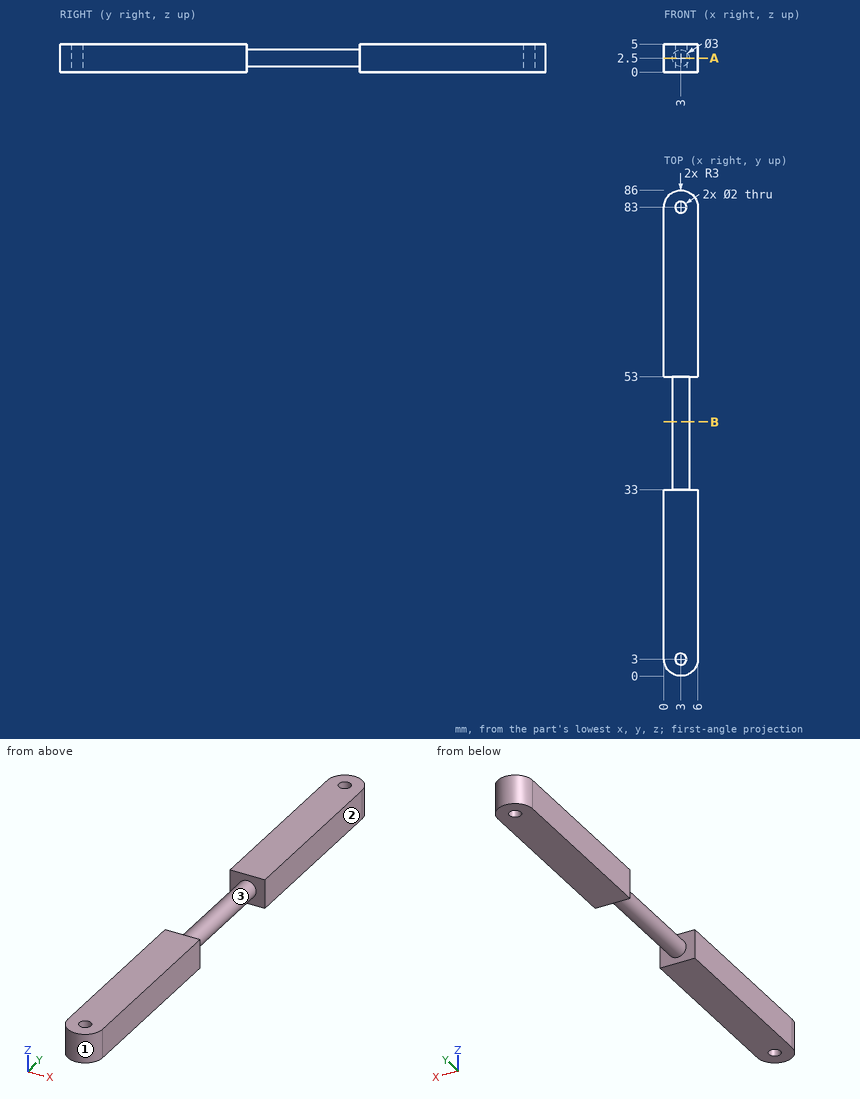
Print and shaded views of the part. All mm, measured from the part's lowest x, y and z. Coordinates: 2 decimals unless noted, no trailing zeros. Loops run counter-clockwise (first coordinate to the right, second up) from the corner with the lowest first, then second, coordinate; pieces in that order, holes last. Notation, with made-up numbers: (46, 62.25) -> (54, 62.25) arc R20 ccw to (54, 72.25) -> close; hole circle Ø9 at (56.25, 14.5). An arc over 180 degrees is marked (long way). Use a Markdown table: item, result. Add a question column.
Item 1: Probe probe 1 along Y at (x, z) = (3, 2.85); probe 2 along Y at (x, z) = (2.9, 4.5); probe 3 along X at (y, z) = (83, 2.15). List the from-to ranges inside material, lowest first.
Item 2: Band-saw the part on B-B on y = 45. Write the cut outline in (x, z), plus the area to 3 significant figures.
Item 3: Flat gauge pins, fed straight in: P1, Ø2, axis at x = 5, z = 2.5, coming from the +Y side; P2, Ø1.5, axis at x = 4, z = 1.5, coming from the -Y side. Where does each tip first touch, or does it go through?
Item 4: Band-saw the part on A-A on z = 2.5. Write the cut outline in (x, y).
Item 5: Pull direction Y, two halves, no side cores. Call the marked faces 1, 2 and 3: +Y half, -Y half, draft (parallel to the pull), parting line (faces both ways), or undercut.
Geometry says:
| question | item | result |
|---|---|---|
| 1 | probe 1 | 0 to 2, 4 to 82, 84 to 86 |
| 1 | probe 2 | 0 to 2.01, 3.99 to 33, 53 to 82.01, 83.99 to 86 |
| 1 | probe 3 | 0 to 2, 4 to 6 |
| 2 | outline | circle Ø3 at (3, 2.5) |
| 2 | area | 7.07 mm² |
| 3 | P1 | y = 85.83 |
| 3 | P2 | y = 0.01 |
| 4 | outline | (0, 3) arc R3 ccw to (6, 3) -> (6, 33) -> (4.5, 33) -> (4.5, 53) -> (6, 53) -> (6, 83) arc R3 ccw to (0, 83) -> (0, 53) -> (1.5, 53) -> (1.5, 33) -> (0, 33) -> close; hole circle Ø2 at (3, 3); hole circle Ø2 at (3, 83) |
| 5 | face 1 | -Y half |
| 5 | face 2 | draft |
| 5 | face 3 | undercut |
